Verification items for the finished model (mm, model axes). A direction names the side the tool comes from. Round coordinates to 2 decimals unless told otherwise and drop trailing zeros. Order: outer loops, then holes, each group sorted by start corner. A loop starts at its lowest first (then second) coordinate and runs counter-clockwise, first axis right, second up. Notation, with made-up numbers: (-18.75, -23) -> (22.25, -23) arc R21 cw to (22.25, -15) -> close; hole circle Ø8 at (-15, -8). An arc over 180 degrees is marked (long way). Put each result on its own line as item: value.
```python
from build123d import *

# Parameters (mm, degrees)
SKETCH1_W           = 15.5
SKETCH1_H           = 11
BOSS_EXTRUDE1_DEPTH = 1.6
BOSS_EXTRUDE2_DEPTH = 1.6
SKETCH3_W           = 15.5
SKETCH3_H           = 2.7
BOSS_EXTRUDE3_DEPTH = 2.7
SKETCH4_W           = 40.2
SKETCH4_H           = 1.6
BOSS_EXTRUDE4_DEPTH = 30
SKETCH5_W           = 30.1
SKETCH5_H           = 9.2
BOSS_EXTRUDE5_DEPTH = 12.1
SKETCH6_R           = 2
CUT_EXTRUDE1_DEPTH  = 2
LPATTERN1_COUNT     = 6
LPATTERN1_PITCH     = 5


with BuildPart() as part:
    # Sketch1 → Boss-Extrude1 (new body)
    with BuildSketch(Plane(origin=(0, 0, 0), x_dir=(1, 0, 0), z_dir=(0, 1, 0))):
        with Locations((7.75, -5.5)):
            Rectangle(SKETCH1_W, SKETCH1_H)
    extrude(amount=BOSS_EXTRUDE1_DEPTH)

    # Sketch2 → Boss-Extrude2 (add, through all)
    with BuildSketch(Plane(origin=(0, 1.6, 0), x_dir=(1, 0, 0), z_dir=(0, 1, 0))):
        with BuildLine():
            Line((-1.75, -4), (-1.75, -2.6))
            ThreePointArc((-1.75, -2.6), (-4.65, -5.5), (-1.75, -8.4))
            Line((-1.75, -8.4), (-1.75, -7))
            ThreePointArc((-1.75, -7), (-3.25, -5.5), (-1.75, -4))
        make_face()
        with BuildLine():
            ThreePointArc((0, -3.187533784), (-0.827002716, -2.750804479), (-1.75, -2.6))
            Line((-1.75, -2.6), (-1.75, -4))
            ThreePointArc((-1.75, -4), (-0.689339828, -4.439339828), (-0.25, -5.5))
            ThreePointArc((-0.25, -5.5), (-0.689339828, -6.560660172), (-1.75, -7))
            Line((-1.75, -7), (-1.75, -8.4))
            ThreePointArc((-1.75, -8.4), (-0.827002716, -8.249195521), (0, -7.812466216))
            Line((0, -7.812466216), (0, -3.187533784))
        make_face()
        with BuildLine():
            Line((0, -2.6), (-1.75, -2.6))
            ThreePointArc((-1.75, -2.6), (-0.827002716, -2.750804479), (0, -3.187533784))
            Line((0, -3.187533784), (0, -2.6))
        make_face()
        with BuildLine():
            ThreePointArc((0, -7.812466216), (-0.827002716, -8.249195521), (-1.75, -8.4))
            Line((-1.75, -8.4), (0, -8.4))
            Line((0, -8.4), (0, -7.812466216))
        make_face()
        with BuildLine():
            ThreePointArc((20.15, -5.5), (19.300609665, -3.449390335), (17.25, -2.6))
            Line((17.25, -2.6), (17.25, -4))
            ThreePointArc((17.25, -4), (18.310660172, -4.439339828), (18.75, -5.5))
            ThreePointArc((18.75, -5.5), (18.310660172, -6.560660172), (17.25, -7))
            Line((17.25, -7), (17.25, -8.4))
            ThreePointArc((17.25, -8.4), (19.300609665, -7.550609665), (20.15, -5.5))
        make_face()
        with BuildLine():
            Line((17.25, -4), (17.25, -2.6))
            ThreePointArc((17.25, -2.6), (16.327002716, -2.750804479), (15.5, -3.187533784))
            Line((15.5, -3.187533784), (15.5, -7.812466216))
            ThreePointArc((15.5, -7.812466216), (16.327002716, -8.249195521), (17.25, -8.4))
            Line((17.25, -8.4), (17.25, -7))
            ThreePointArc((17.25, -7), (15.75, -5.5), (17.25, -4))
        make_face()
        with BuildLine():
            Line((17.25, -2.6), (15.5, -2.6))
            Line((15.5, -2.6), (15.5, -3.187533784))
            ThreePointArc((15.5, -3.187533784), (16.327002716, -2.750804479), (17.25, -2.6))
        make_face()
        with BuildLine():
            Line((15.5, -7.812466216), (15.5, -8.4))
            Line((15.5, -8.4), (17.25, -8.4))
            ThreePointArc((17.25, -8.4), (16.327002716, -8.249195521), (15.5, -7.812466216))
        make_face()
    extrude(amount=-BOSS_EXTRUDE2_DEPTH)

    # Sketch3 → Boss-Extrude3 (add)
    with BuildSketch(Plane(origin=(0, 1.6, 0), x_dir=(1, 0, 0), z_dir=(0, 1, 0))):
        with Locations((7.75, -9.15)):
            Rectangle(SKETCH3_W, SKETCH3_H)
    extrude(amount=BOSS_EXTRUDE3_DEPTH)

    # Sketch4 → Boss-Extrude4 (add)
    with BuildSketch(Plane(origin=(0, 4.3, 0), x_dir=(1, 0, 0), z_dir=(0, 1, 0))):
        with Locations((7.75, -10.112281479)):
            Rectangle(SKETCH4_W, SKETCH4_H)
    extrude(amount=BOSS_EXTRUDE4_DEPTH)

    # Sketch5 → Boss-Extrude5 (add)
    with BuildSketch(Plane(origin=(0, 0, 9.312281479), x_dir=(-1, 0, 0), z_dir=(0, 0, -1))):
        with Locations((-6.7, 27.4)):
            Rectangle(SKETCH5_W, SKETCH5_H)
    extrude(amount=BOSS_EXTRUDE5_DEPTH)

    # Sketch6 → Cut-Extrude1 (cut)
    with BuildSketch(Plane(origin=(0, 0, -2.787718521), x_dir=(-1, 0, 0), z_dir=(0, 0, -1))):
        with Locations((-19.35, 27.8)):
            Circle(SKETCH6_R)
    cut_extrude1 = extrude(amount=-CUT_EXTRUDE1_DEPTH, mode=Mode.SUBTRACT)

    # LPattern1: Cut-Extrude1 ×6
    with Locations(*[(-i * LPATTERN1_PITCH, 0, 0) for i in range(1, LPATTERN1_COUNT)]):
        add(cut_extrude1, mode=Mode.SUBTRACT)


solid = part.part
```
Item 1: Sectioned sample at C-C, the plane z = 3.25. Record the boundary of the cut face in (x, y), then the cut area to 3 significant figures.
Geometry check:
outline: (-8.35, 22.8) -> (21.75, 22.8) -> (21.75, 32) -> (-8.35, 32) -> close; (-3.58, 0) -> (19.08, 0) -> (19.08, 1.6) -> (-3.58, 1.6) -> close
area: 313 mm2
Item 2: Tool access check on faces 4 (the face through (16, 1, 2.6)), 5 (the face through (-4.65, 0.81, 5.44)), 6 (the face through (4, 28, -0.788)), 7 (the face through (-1, 1, 8.4)), 8 (the face through (8, 4.3, 9)). Record the directions out of +Z, -Z, +X, -X, +Y, -Y that give a thin tool (end or side, any length) a straight path to the whole face; none if there is none.
Geometry check:
face 4: -Z, +X, -Y
face 5: -X, -Y
face 6: -Z
face 7: +Z, -X, -Y
face 8: -Z, +X, -X
Item 3: Depth check by flat-ended pin: pin 1 Ø4.5 at (x, y) = (4.35, 27.8) entering from +Z; pin 2 Ø1 at (x, z) = (-7, 0) entering from +Y; pin 3 Ø1.3 at (x, y) = (-1, 1) entering from -Z. Enter the tip coordinate at first touch or a pass-through.
Geometry check:
pin 1: z = 10.91
pin 2: y = 32
pin 3: z = 2.6
Item 4: Sectioned sample at A-A, the plane x = 19.35. Record the boundary of the cut face in (y, z).
Geometry check:
outline: (0, 3.5) -> (1.6, 3.5) -> (1.6, 7.5) -> (0, 7.5) -> close; (4.3, 9.31) -> (22.8, 9.31) -> (22.8, -2.79) -> (25.8, -2.79) -> (25.8, -0.79) -> (29.8, -0.79) -> (29.8, -2.79) -> (32, -2.79) -> (32, 9.31) -> (34.3, 9.31) -> (34.3, 10.91) -> (4.3, 10.91) -> close
Item 5: Release check for a two-part mould opening along Y. For faces 1 (the face through (-0.39, 29.783, -1.802)), 2 (the face through (7, 34.3, 10)), 3 (the face through (27.85, 19, 10)) record: pulls with the +Y half, pulls with the -Y half, needs draft (parallel to the pull), parting line crosses it, or undercut.
Geometry check:
face 1: undercut
face 2: pulls with the +Y half
face 3: needs draft
Item 6: Material ranges on line 1 along Y through (x, z) = (9.35, -1.6); line 2 along Y through (x, z) = (0, 6); line 3 along Y through (x, z) = (-1.5, 4.75), recorded low to high.
Geometry check:
line 1: 22.8 to 25.8, 29.8 to 32
line 2: 0 to 1.6, 22.8 to 32
line 3: 22.8 to 32
Item 7: Sectioned sample at D-D, the plane x = 14.35. Record the boundary of the cut face in (y, z), then the cut area to 3 significant figures.
Geometry check:
outline: (0, 0) -> (1.6, 0) -> (1.6, 7.8) -> (4.3, 7.8) -> (4.3, 9.31) -> (22.8, 9.31) -> (22.8, -2.79) -> (25.8, -2.79) -> (25.8, -0.79) -> (29.8, -0.79) -> (29.8, -2.79) -> (32, -2.79) -> (32, 9.31) -> (34.3, 9.31) -> (34.3, 10.91) -> (4.3, 10.91) -> (4.3, 10.5) -> (1.6, 10.5) -> (1.6, 11) -> (0, 11) -> close
area: 176 mm2
